Part model, mm, in its own coordinate system. Give positions to 0.01 mm unless a question says otherwise; leave off trailing zeros. Order: outer loops, then holes, each group sorted by start corner. A loop starts at its lowest first (then second) coordinate and runs counter-clockwise, first axis right, second up. Notation, with made-up numbers: M 80,-5.5 L 89,-5.5 A20 cw 89,29.5 Z; hole C -1,45 d6. An arc over 180 degrees is marked long. One line per question, with ' | ' between items.
```python
from build123d import *

# Parameters (mm, degrees)
SKETCH1_W           = 14
SKETCH1_H           = 200
BOSS_EXTRUDE1_DEPTH = 1
SKETCH2_R           = 2.5
BOSS_EXTRUDE2_DEPTH = 1


with BuildPart() as part:
    # Sketch1 → Boss-Extrude1 (new body)
    with BuildSketch(Plane(origin=(0, 0, 0), x_dir=(1, 0, 0), z_dir=(0, 1, 0))):
        with Locations((7, 100)):
            Rectangle(SKETCH1_W, SKETCH1_H)
    extrude(amount=BOSS_EXTRUDE1_DEPTH)

    # Sketch2 → Boss-Extrude2 (add)
    with BuildSketch(Plane.XZ):
        with BuildLine():
            Line((0, -200), (14, -200))
            Line((14, -200), (14, -213))
            ThreePointArc((14, -213), (7, -220), (0, -213))
            Line((0, -213), (0, -200))
        make_face()
        with Locations(Location((7, -213, 0), (0, 0, 270))):
            Circle(SKETCH2_R, mode=Mode.SUBTRACT)
    extrude(amount=-BOSS_EXTRUDE2_DEPTH)


solid = part.part
```
1. Slice it at A-A on x = 7. Give the cut face in (y, z).
Worked out:
outline: M 0,-220 L 1,-220 L 1,-215.5 L 0,-215.5 Z; M 0,-210.5 L 1,-210.5 L 1,0 L 0,0 Z
2. Mould opens along Z. For faces 1 (the flat face through (7, 1, -108)), 2 (the cylindrical face through (7.15, 0.49, -220)), 3 (the cylindrical face through (6.04, 0.49, -215.31)) say: released by +Z, released by -Z, zero draft, split by the parting line, or undercut.
Worked out:
face 1: zero draft | face 2: released by -Z | face 3: undercut
3. Probe L1, parallel to X at y = 0.3, z = -213; L2, parallel to Z at x = 6, y = 0.5; L3, parallel to Z at x = 4, y = 0.25. List the from-to ranges inside material, lowest first. Write a range as from..to.
Worked out:
L1: x = 0..4.5, 9.5..14 | L2: z = -219.93..-215.29, -210.71..0 | L3: z = -219.32..0
